For this review, take the finished solid that the model builds, in its own axes (mm). Coordinates: 2 decimals unless noted, no trailing zeros. Loops run counter-clockwise (first coordinate to the right, second up) from the corner with the lowest first, then second, coordinate; pieces in that order, holes last. Notation, with made-up numbers: M -24.75,34.25 L 19.25,34.25 A21 ccw 19.25,55.25 Z; hole C -7,-15 d10. An arc over 180 degrees is marked long. Answer as a JSON object with one key per item and string values. Group by question number.
Item 1: Add section B-B (y = 15). State the section outline as (x, z) points (1 decimal).
Item 2: Wall thickness on L1, parallel to Z at x = 0, y = 20; L2, parallel to Y at x = 0, z = 7.75; L3, parallel to Z at x = -2, y = 3.5: over which ranges is each line inside the solid? List them lowest first. Write a range as from..to.
Item 3: Mouldability with a two-part tool opening along X and no side actions: class faces 1 (the face through (-4.77, 14.79, -1.5)), 2 (the face through (7.18, 0.25, -4.06)), 3 (the face through (2.2, 14.8, 8.5)) as +X half, -X half, draft (parallel to the pull), parting line (faces both ways), or undercut.
Item 4: Insertion check: pin 1 (1 mm diameter, centred on y = 21.5, z = 4, fed in from -X); pin 2 (5 mm diameter, centred on y = 11, z = 5.5, fed in from -X); pin 3 (6 mm diameter, centred on y = 5.5, z = 4.5, fed in from +X). Each pin has a flat end and moves straight along its axis. Give the tip position at first contact, or say it passes through.
Item 5: Add section A-A (x = 4). State the section outline as (y, z) points, then the cut area to 4 significant figures.
Item 6: Add section D-D (z = -4). State the section outline as (x, y) points.
Item 7: Add section C-C (x = 0). State the section outline as (y, z) points, then the cut area to 4 significant figures.
Autodesk Inventor part; units mm, degrees
ref_plane "YZ Plane" through (0, 0, 0) normal (1, 0, 0) x (0, 1, 0)
ref_plane "XZ Plane" through (0, 0, 0) normal (0, 1, 0) x (-1, 0, 0)
ref_plane "XY Plane" through (0, 0, 0) normal (0, 0, 1) x (1, 0, 0)
sketch "Sketch1" plane through (0, 0, 0) normal (0, 1, 0) x (-1, 0, 0)
  circle A0 centre (0, 0) radius 5
  line L0 (9.815, 0) -> (4.9075, -8.5)
  line L1 (4.9075, -8.5) -> (-4.9075, -8.5)
  line L2 (-4.9075, -8.5) -> (-9.815, 0)
  line L3 (-9.815, 0) -> (-4.9075, 8.5)
  line L4 (-4.9075, 8.5) -> (4.9075, 8.5)
  line L5 (4.9075, 8.5) -> (9.815, 0)
  dimension "d0" = 10
  dimension "d1" = 17
extrude "Extrusion1" add sketch "Sketch1" along normal blind 30
chamfer "Chamfer1" distance 0.5 angle 45 12 edges at (7.3612, 0, 4.25) (0, 0, 8.5) (-7.3612, 0, 4.25) (-7.3612, 0, -4.25) (0, 0, -8.5) (7.3612, 0, -4.25) (7.3612, 30, -4.25) (7.3612, 30, 4.25) (0, 30, 8.5) (-7.3612, 30, 4.25) (-7.3612, 30, -4.25) (0, 30, -8.5)
thread "Thread1"
sketch "Sketch2" plane through (-4.9075, 29.5, 8.5) normal (0, 0, 1) x (1, 0, 0)
  circle A0 centre (4.9075, -14.5) radius 2
  point P0 (4.9075, -29.5)
  dimension "d9" = 4
  dimension "d10" = 15
extrude "Extrusion2" cut sketch "Sketch2" against normal blind 26.75
thread "Thread2"
thread "Thread3"
properties part number "КВ33.000.105 - Каретка" material "Iron, Cast"
From the geometry:
{
 "1": {"outline": "M -9.8,0 L -4.9,-8.5 L -2,-8.5 L -2,-4.6 A5 cw -2,4.6 L -2,8.5 L -4.9,8.5 Z; M 2,-8.5 L 4.9,-8.5 L 9.8,0 L 4.9,8.5 L 2,8.5 L 2,4.6 A5 cw 2,-4.6 Z"},
 "2": {"L1": "z = -8.5..-5, 5..8.5", "L2": "y = 0..13, 17..30", "L3": "z = -8.5..-4.58, 4.58..8.5"},
 "3": {"face 1": "undercut", "face 2": "+X half", "face 3": "draft"},
 "4": {"pin 1": "stops at x = -7.79", "pin 2": "stops at x = -8.08", "pin 3": "stops at x = 8.95"},
 "5": {"outline": "M 0,-8 L 0.5,-8.5 L 29.5,-8.5 L 30,-8 L 30,-3 L 0,-3 Z; M 0,3 L 30,3 L 30,8 L 29.5,8.5 L 0.5,8.5 L 0,8 Z", "area": "329.5 mm²"},
 "6": {"outline": "M -7.51,0.5 L -6.93,0 L -3,0 L -3,30 L -6.93,30 L -7.51,29.5 Z; M 3,0 L 6.93,0 L 7.51,0.5 L 7.51,29.5 L 6.93,30 L 3,30 Z"},
 "7": {"outline": "M 0,-8 L 0.5,-8.5 L 13,-8.5 L 13,-5 L 0,-5 Z; M 0,5 L 13,5 L 13,8.5 L 0.5,8.5 L 0,8 Z; M 17,-8.5 L 29.5,-8.5 L 30,-8 L 30,-5 L 17,-5 Z; M 17,5 L 30,5 L 30,8 L 29.5,8.5 L 17,8.5 Z", "area": "181.5 mm²"}
}
